Could you check a few things on this drawing? It's one solid part, dimensions in mm from its lowest x, y, z. A direction names the side the tool comes from. Give positions to 0.01 mm unless a question says otherwise; leave off trailing zeros. Order: outer loops, then holes, each group sorted by start corner. A loop starts at its lowest first (then second) coordinate and runs counter-clockwise, first axis right, second up. Notation, with made-up numbers: (-17, 37.5) -> (32, 37.5) arc R19 ccw to (32, 50.5) -> close; hole circle Ø9 at (39.25, 39.5). An arc over 180 degrees is marked (long way). Answer as a JSON object with one key per item and string values.
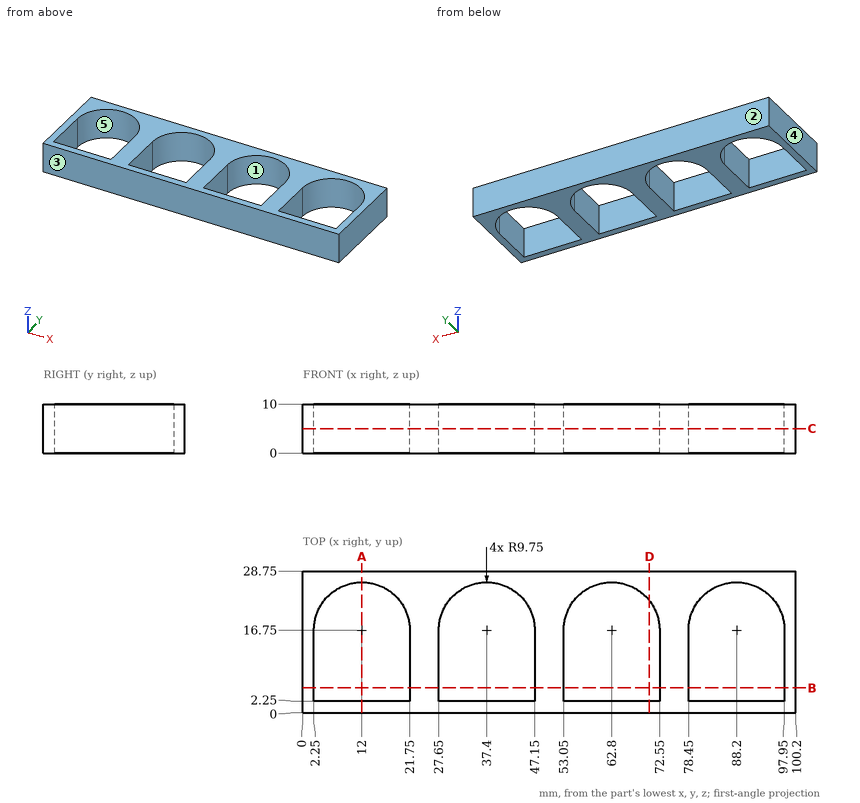
1. If we section it at C-C on z = 5: Please give me the cut outline in (x, y).
Worked answers:
{"outline": "(0, 0) -> (100.2, 0) -> (100.2, 28.75) -> (0, 28.75) -> close; hole (2.25, 2.25) -> (21.75, 2.25) -> (21.75, 16.75) arc R9.75 ccw to (2.25, 16.75) -> close; hole (27.65, 2.25) -> (47.15, 2.25) -> (47.15, 16.75) arc R9.75 ccw to (27.65, 16.75) -> close; hole (53.05, 2.25) -> (72.55, 2.25) -> (72.55, 16.75) arc R9.75 ccw to (53.05, 16.75) -> close; hole (78.45, 2.25) -> (97.95, 2.25) -> (97.95, 16.75) arc R9.75 ccw to (78.45, 16.75) -> close"}
2. Please list where these lines run through material, in increasing order: L1, parallel to X at y = 12.75, z = 8.5; L2, parallel to X at y = 20.5, z = 7; L3, parallel to Y at x = 43, z = 8.5.
Worked answers:
{"L1": "0 to 2.25, 21.75 to 27.65, 47.15 to 53.05, 72.55 to 78.45, 97.95 to 100.2", "L2": "0 to 3, 21 to 28.4, 46.4 to 53.8, 71.8 to 79.2, 97.2 to 100.2", "L3": "0 to 2.25, 24.73 to 28.75"}
3. If we mould it in two halves opening along Y, with no side actions, what happens to the marked faces 1, 2 and 3? For each: +Y half, -Y half, draft (parallel to the pull), parting line (faces both ways), or undercut.
Worked answers:
{"face 1": "undercut", "face 2": "+Y half", "face 3": "-Y half"}
4. If we section it at D-D on x = 70.5: Please give me the cut outline in (y, z).
Worked answers:
{"outline": "(0, 0) -> (2.25, 0) -> (2.25, 10) -> (0, 10) -> close; (22.73, 0) -> (28.75, 0) -> (28.75, 10) -> (22.73, 10) -> close"}
5. If we section it at B-B on y = 5: Please give me the cut outline in (x, z), then the cut area to 3 significant figures.
Worked answers:
{"outline": "(0, 0) -> (2.25, 0) -> (2.25, 10) -> (0, 10) -> close; (21.75, 0) -> (27.65, 0) -> (27.65, 10) -> (21.75, 10) -> close; (47.15, 0) -> (53.05, 0) -> (53.05, 10) -> (47.15, 10) -> close; (72.55, 0) -> (78.45, 0) -> (78.45, 10) -> (72.55, 10) -> close; (97.95, 0) -> (100.2, 0) -> (100.2, 10) -> (97.95, 10) -> close", "area": "222 mm²"}
6. For the marked faces 4 and 5, which set-ups out of +Z, -Z, +X, -X, +Y, -Y let a thin tool reach every point of the face, with its end or its side?
Worked answers:
{"face 4": "+Z, -Z, -X, +Y, -Y", "face 5": "+Z, -Z"}
7. If we section it at A-A on x = 12: Please give me the cut outline in (y, z), then the cut area to 3 significant figures.
Worked answers:
{"outline": "(0, 0) -> (2.25, 0) -> (2.25, 10) -> (0, 10) -> close; (26.5, 0) -> (28.75, 0) -> (28.75, 10) -> (26.5, 10) -> close", "area": "45.0 mm²"}
